from build123d import *

# Parameters (mm, degrees)
SKETCH1_R           = 4.625
BOSS_EXTRUDE1_DEPTH = 0.845
SKETCH2_R           = 6.035
BOSS_EXTRUDE2_DEPTH = 1.06
SKETCH3_R           = 6.035
BOSS_EXTRUDE3_DEPTH = 1.06
BOSS_EXTRUDE4_DEPTH = 2
BOSS_EXTRUDE5_DEPTH = 2
SKETCH6_R           = 3.5306
CUT_EXTRUDE1_DEPTH  = 8.81


with BuildPart() as part:
    # Sketch1 → Boss-Extrude1 (new body, symmetric)
    with BuildSketch(Plane(origin=(0, 0, 0), x_dir=(1, 0, 0), z_dir=(0, 1, 0))):
        Circle(SKETCH1_R)
    extrude(amount=BOSS_EXTRUDE1_DEPTH, both=True)

    # Sketch2 → Boss-Extrude2 (add)
    with BuildSketch(Plane(origin=(0, 0.845, 0), x_dir=(1, 0, 0), z_dir=(0, 1, 0))):
        Circle(SKETCH2_R)
    extrude(amount=BOSS_EXTRUDE2_DEPTH)

    # Sketch3 → Boss-Extrude3 (add)
    with BuildSketch(Plane.XZ.offset(0.845)):
        Circle(SKETCH3_R)
    extrude(amount=BOSS_EXTRUDE3_DEPTH)

    # Sketch4 → Boss-Extrude4 (add)
    with BuildSketch(Plane(origin=(0, 1.905, 0), x_dir=(1, 0, 0), z_dir=(0, 1, 0))):
        with BuildLine():
            Line((-3.881348315, 1.892157303), (-3.881348315, 0))
            Line((-3.881348315, 0), (-3.881348315, -1.892157303))
            ThreePointArc((-3.881348315, -1.892157303), (0, -4.318), (3.881348315, -1.892157303))
            Line((3.881348315, -1.892157303), (3.881348315, 0))
            Line((3.881348315, 0), (3.881348315, 1.892157303))
            ThreePointArc((3.881348315, 1.892157303), (0, 4.318), (-3.881348315, 1.892157303))
        make_face()
    extrude(amount=BOSS_EXTRUDE4_DEPTH)

    # Sketch5 → Boss-Extrude5 (add)
    with BuildSketch(Plane.XZ.offset(1.905)):
        with BuildLine():
            Line((-4.024811429, 2.569713604), (-4.024811429, 0))
            Line((-4.024811429, 0), (-4.024811429, -2.569713604))
            ThreePointArc((-4.024811429, -2.569713604), (0, -4.7752), (4.024811429, -2.569713604))
            Line((4.024811429, -2.569713604), (4.024811429, 0))
            Line((4.024811429, 0), (4.024811429, 2.569713604))
            ThreePointArc((4.024811429, 2.569713604), (0, 4.7752), (-4.024811429, 2.569713604))
        make_face()
    extrude(amount=BOSS_EXTRUDE5_DEPTH)

    # Sketch6 → Cut-Extrude1 (cut, through all)
    with BuildSketch(Plane(origin=(0, 3.905, 0), x_dir=(1, 0, 0), z_dir=(0, 1, 0))):
        Circle(SKETCH6_R)
    extrude(amount=-CUT_EXTRUDE1_DEPTH, mode=Mode.SUBTRACT)


solid = part.part
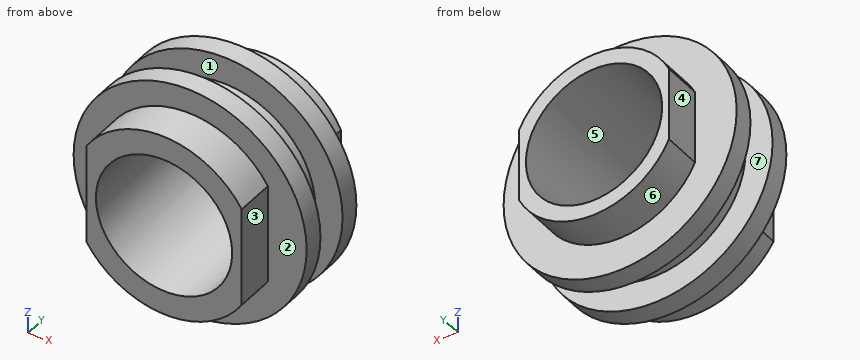
Model file for the job. Use its own axes, mm. Face numbers are marked on the shaded views. A direction names the side the tool comes from. Round coordinates to 2 decimals unless told otherwise and drop trailing zeros. Loops run counter-clockwise (first coordinate to the right, second up) from the corner with the lowest first, then second, coordinate; pieces in that order, holes last. Notation, with made-up numbers: (-21, 80) - (26, 80) arc R21 cw to (26, 111) - close; hole circle Ø10 at (50, 0.25). An arc over 180 degrees is marked (long way). Write each question's results on one line, items separated by ' | '.
(1) Saw through at D-D, the plane y = -1.5. List the corners of the cut face in (x, z) (3 decimals).
Answer below:
outline: circle Ø12.07 at (0, 0); hole circle Ø7.061 at (0, 0)
(2) Wall check: L1, parallel to Z at x = 0, y = 1 (3 decimals); L2, parallel to Y at x = 5, z = -2.5 (3 decimals); L3, parallel to Z at x = 0, y = 0 (3 decimals). Give the ranges that are in metal, low to high.
Answer below:
L1: z = -6.035 to -3.531, 3.531 to 6.035 | L2: y = -1.905 to -0.845, 0.845 to 1.905 | L3: z = -4.625 to -3.531, 3.531 to 4.625
(3) 3-axis set-ups, long thin cutter, end or side, ignore diameter. For the marked faces 1, 2, 3 and 4: which of +Z, -Z, +X, -X, +Y, -Y reach the whole face in a straight line?
Answer below:
face 1: none | face 2: -Y | face 3: +Z, -Z, +X, -Y | face 4: +Z, -Z, -X, +Y
(4) Saw through at B-B, the plane y = 2.75. List the corners of the cut face in (x, z), then the cut area to 3 significant figures.
Answer below:
outline: (-3.88, -1.89) arc R4.32 ccw to (3.88, -1.89) - (3.88, 1.89) arc R4.32 ccw to (-3.88, 1.89) - close; hole circle Ø7.06 at (0, 0) | area: 17.2 mm^2
(5) Saw through at A-A, the plane z = 0. List the corners of the cut face in (x, y) (3 decimals).
Answer below:
outline: (-6.035, -1.905) - (-4.025, -1.905) - (-4.025, -3.905) - (-3.531, -3.905) - (-3.531, 3.905) - (-3.881, 3.905) - (-3.881, 1.905) - (-6.035, 1.905) - (-6.035, 0.845) - (-4.625, 0.845) - (-4.625, -0.845) - (-6.035, -0.845) - close; (3.531, -3.905) - (4.025, -3.905) - (4.025, -1.905) - (6.035, -1.905) - (6.035, -0.845) - (4.625, -0.845) - (4.625, 0.845) - (6.035, 0.845) - (6.035, 1.905) - (3.881, 1.905) - (3.881, 3.905) - (3.531, 3.905) - close
(6) Saw through at C-C, the plane x = -1.5. List the corners of the cut face in (y, z) (1 decimal), then the cut area to 3 significant figures.
Answer below:
outline: (-3.9, -4.5) - (-1.9, -4.5) - (-1.9, -5.8) - (-0.8, -5.8) - (-0.8, -4.4) - (0.8, -4.4) - (0.8, -5.8) - (1.9, -5.8) - (1.9, -4) - (3.9, -4) - (3.9, -3.2) - (-3.9, -3.2) - close; (-3.9, 3.2) - (3.9, 3.2) - (3.9, 4) - (1.9, 4) - (1.9, 5.8) - (0.8, 5.8) - (0.8, 4.4) - (-0.8, 4.4) - (-0.8, 5.8) - (-1.9, 5.8) - (-1.9, 4.5) - (-3.9, 4.5) - close | area: 24.0 mm^2
(7) Mould opens along Z. For the marked faces 5, 6 and 7 say: released by +Z, released by -Z, zero draft, split by the parting line, or undercut.
Answer below:
face 5: undercut | face 6: released by -Z | face 7: zero draft
(8) Pin check, flat tips, straight feed: pin 1 (5 mm diameter, centred on x = -2.5, z = -2, fed in from +Y) (3 decimals); pin 2 (1.5 mm diameter, centred on x = -3.5, z = 4.5, fed in from +Y) (3 decimals); pin 3 (1.6 mm diameter, centred on y = 3, z = 0, fed in from -X); pin 4 (1.6 mm diameter, centred on y = -3.5, z = -0.5, fed in from -X). Stop position of each tip, or through.
Answer below:
pin 1: stops at y = 3.905 | pin 2: stops at y = 1.905 | pin 3: stops at x = -3.88 | pin 4: stops at x = -4.02
